Part model, mm, in its own coordinate system. Face numbers are marked on the shaded views. A direction names the side the tool comes from. Give positions to 0.01 mm unless a question says otherwise; leave off trailing zeros. Order: outer loops, then holes, each group sorted by start corner. A loop starts at its lowest first (then second) coordinate and runs counter-clockwise, first axis right, second up. Notation, with made-up numbers: (71, 88.25) -> (102, 88.25) arc R25 cw to (102, 105.25) -> close; hole circle Ø2 at (84, 78). An arc over 180 degrees is marked (long way). Write item = value, one per line. Start each with the question number.
(1) Flat gauge pins, fed straight in: pin 1 (2 mm diameter, centred on x = -2, y = 12.5, fed in from -Z); pin 2 (1 mm diameter, centred on x = 2, y = -2, fed in from +Z); pin 3 (2 mm diameter, centred on x = -3, y = 2, fed in from +Z). Where does each tip first touch, or does it go through?
(2) Probe line 1 along Y through (x, z) = (2.25, 22.5); line 2 along Y through (x, z) = (0, 29); line 3 along Y through (x, z) = (0, 21). List the from-to ranges inside material, lowest first. Write a range as from..to.
(3) Saw through at C-C, the plane y = 21. List the corners of the cut face in (x, z).
(4) Saw through at D-D, the plane z = 9. List the corners of the cut face in (x, y).
(5) Which spindle directions (+Z, -Z, +X, -X, +Y, -Y) get a long thin tool onto all of the face, cutting with end or side? Do the marked faces 1 and 2. Say none if no direction does.
(6) Saw through at B-B, the plane x = 0. List the corners of the cut face in (y, z), then the cut area to 3 significant figures.
(7) Saw through at A-A, the plane z = 18. List the corners of the cut face in (x, y).
(8) Two-plate mould, pull along Y, no slides. Class the marked faces 3, 4 and 5: pulls with the +Y half, pulls with the -Y half, needs draft (parallel to the pull), parting line crosses it, or undercut.
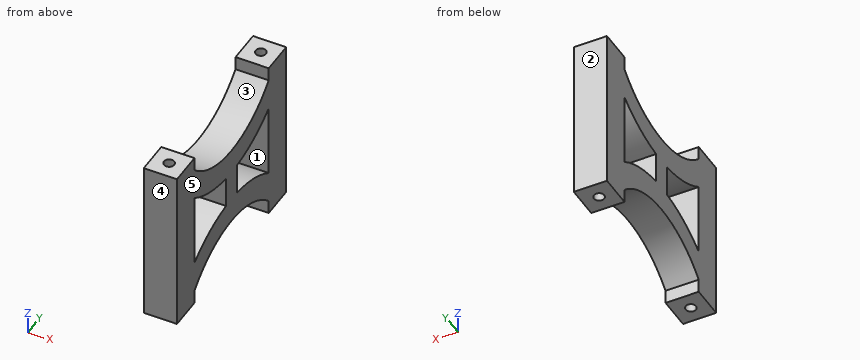
from build123d import *

# Parameters (mm, degrees)
SKETCH1_W             = 8
SKETCH1_H             = 8
SKETCH1_R             = 1.25
BOSS_EXTRUDE1_DEPTH   = 40
BOSS_EXTRUDE1_2_DEPTH = 40
BOSS_EXTRUDE2_DEPTH   = 8


with BuildPart() as part:
    # Sketch1 → Boss-Extrude1 (new body)
    with BuildSketch(Plane.XY):
        with Locations((0, 21)):
            Rectangle(SKETCH1_W, SKETCH1_H)
        with Locations((0, 21)):
            Circle(SKETCH1_R, mode=Mode.SUBTRACT)
    extrude(amount=BOSS_EXTRUDE1_DEPTH)



with BuildPart() as body_2:
    # Sketch1 → Boss-Extrude1 2 (new body)
    with BuildSketch(Plane.XY):
        with Locations((0, -21)):
            Rectangle(SKETCH1_W, SKETCH1_H)
        with Locations(Location((0, -21, 0), (0, 0, 180))):
            Circle(SKETCH1_R, mode=Mode.SUBTRACT)
    extrude(amount=BOSS_EXTRUDE1_2_DEPTH)


with BuildPart() as part_1:
    add(part.part)

    add(body_2.part)  # Boss-Extrude2 merges body 2
    # Sketch2 → Boss-Extrude2 (add)
    with BuildSketch(Plane.ZY.offset(4)):
        with BuildLine():
            Line((3.329640508, 17), (11.063985021, 17))
            ThreePointArc((11.063985021, 17), (14.56966913, 10.077818269), (16.196928044, 2.491089763))
            Line((16.196928044, 2.491089763), (23.803071956, 2.491089763))
            ThreePointArc((23.803071956, 2.491089763), (25.43033087, 10.077818269), (28.936014979, 17))
            Line((28.936014979, 17), (36.670359492, 17))
            ThreePointArc((36.670359492, 17), (29.700211914, 0), (36.670359492, -17))
            Line((36.670359492, -17), (28.936014979, -17))
            ThreePointArc((28.936014979, -17), (25.433314102, -10.086246784), (23.804551435, -2.508910237))
            Line((23.804551435, -2.508910237), (16.195448565, -2.508910237))
            ThreePointArc((16.195448565, -2.508910237), (14.566685898, -10.086246784), (11.063985021, -17))
            Line((11.063985021, -17), (3.329640508, -17))
            ThreePointArc((3.329640508, -17), (10.299788086, 0), (3.329640508, 17))
        make_face()
    extrude(amount=-BOSS_EXTRUDE2_DEPTH)


solid = part_1.part
Results list:
q1.pin_1 = 6.19
q1.pin_2 = 29.83
q1.pin_3 = 29.89
q2.line_1 = -25..-17, -2.51..2.49, 17..25
q2.line_2 = -25..-22.25, -19.75..19.75, 22.25..25
q2.line_3 = -25..-22.25, -19.75..-17, -2.51..2.49, 17..19.75, 22.25..25
q3.outline = (-4, 0) -> (-1.25, 0) -> (-1.25, 40) -> (-4, 40) -> close; (1.25, 0) -> (4, 0) -> (4, 40) -> (1.25, 40) -> close
q4.outline = (-4, -25) -> (4, -25) -> (4, -7.83) -> (-4, -7.83) -> close; (-4, 7.83) -> (4, 7.83) -> (4, 25) -> (-4, 25) -> close; hole circle Ø2.5 at (0, -21); hole circle Ø2.5 at (0, 21)
q5.face_1 = +X, -X
q5.face_2 = +Z, -Z, +X, -X, +Y
q6.outline = (-25, 0) -> (-22.25, 0) -> (-22.25, 40) -> (-25, 40) -> close; (-19.75, 0) -> (-17, 0) -> (-17, 3.33) arc R24.22 cw to (17, 3.33) -> (17, 0) -> (19.75, 0) -> (19.75, 40) -> (17, 40) -> (17, 36.67) arc R24.22 cw to (-17, 36.67) -> (-17, 40) -> (-19.75, 40) -> close; (22.25, 0) -> (25, 0) -> (25, 40) -> (22.25, 40) -> close; hole (-17, 11.06) arc R30.22 cw to (-2.51, 16.2) -> (-2.51, 23.8) arc R30.22 cw to (-17, 28.94) -> close; hole (2.49, 16.2) arc R30.22 cw to (17, 11.06) -> (17, 28.94) arc R30.22 cw to (2.49, 23.8) -> close
q6.area = 919 mm^2
q7.outline = (-4, -25) -> (4, -25) -> (4, -17) -> (-4, -17) -> close; (-4, -2.51) -> (4, -2.51) -> (4, 2.49) -> (-4, 2.49) -> close; (-4, 17) -> (4, 17) -> (4, 25) -> (-4, 25) -> close; hole circle Ø2.5 at (0, -21); hole circle Ø2.5 at (0, 21)
q8.face_3 = undercut
q8.face_4 = pulls with the -Y half
q8.face_5 = needs draft
